```python
from build123d import *

# Parameters (mm, degrees)
PAD_DEPTH       = 28.5
SKETCH001_R     = 14.25
POCKET_DEPTH    = 18.5
SKETCH002_R     = 1.375
POCKET001_DEPTH = 12
SKETCH003_W     = 4
SKETCH003_H     = 10.5
POCKET002_DEPTH = 8
SKETCH004_R     = 1.75
POCKET003_DEPTH = 8
SKETCH005_R     = 3.25
POCKET004_DEPTH = 6
SKETCH006_R     = 1.375
POCKET005_DEPTH = 10
SKETCH007_R     = 1.375
POCKET006_DEPTH = 10


with BuildPart() as recess_pocket:
    # Sketch → Pad (new body)
    with BuildSketch(Plane.YZ):
        with BuildLine():
            ThreePointArc((2.722222, 19.699888), (-1.166667, 20.799832), (-3.5, 17.5))
            Line((-3.5, 17.5), (-3.5, -17.5))
            ThreePointArc((-3.5, -17.5), (-1.166657, -20.799835), (2.722235, -19.699872))
            Line((2.722235, -19.699872), (4.5, -17.5))
            Line((4.5, 17.5), (4.5, -17.5))
            Line((4.5, 17.5), (2.722222, 19.699888))
        make_face()
    extrude(amount=PAD_DEPTH)

    # Sketch001 → Pocket (cut)
    with BuildSketch(Plane.YZ.offset(28.5)):
        Circle(SKETCH001_R)
    extrude(amount=-POCKET_DEPTH, mode=Mode.SUBTRACT)

    # Sketch002 → Pocket001 (cut)
    with BuildSketch(Plane.YZ.offset(28.5)):
        with Locations((0, -17.5)):
            Circle(SKETCH002_R)
        with Locations((0, 17.5)):
            Circle(SKETCH002_R)
    extrude(amount=-POCKET001_DEPTH, mode=Mode.SUBTRACT)

    # Sketch003 → Pocket002 (cut)
    with BuildSketch(Plane(origin=(0, -3.5, 0), x_dir=(0, 0, -1), z_dir=(0, -1, 0))):
        with Locations((-20, 5.25)):
            Rectangle(SKETCH003_W, SKETCH003_H)
        with Locations((20, 5.25)):
            Rectangle(SKETCH003_W, SKETCH003_H)
    extrude(amount=-POCKET002_DEPTH, mode=Mode.SUBTRACT)


with BuildPart() as bottom_screw_hole_pocket:
    # Part__Mirroring: instance of recess-pocket
    add(recess_pocket.part.mirror(Plane(origin=(0, 0, 0), x_dir=(0, -1, 0), z_dir=(1, 0, 0))))

    # Fusion: union recess-pocket
    add(recess_pocket.part)

    # Sketch004 → Pocket003 (cut)
    with BuildSketch(Plane.XZ.offset(3.5)):
        Circle(SKETCH004_R)
    extrude(amount=-POCKET003_DEPTH, mode=Mode.SUBTRACT)

    # Sketch005 → Pocket004 (cut)
    with BuildSketch(Plane.XZ.offset(3.5)):
        Circle(SKETCH005_R)
    extrude(amount=-POCKET004_DEPTH, mode=Mode.SUBTRACT)

    # Sketch006 → Pocket005 (cut)
    with BuildSketch(Plane.XY.offset(18)):
        with Locations((0, 0.5)):
            Circle(SKETCH006_R)
    extrude(amount=-POCKET005_DEPTH, mode=Mode.SUBTRACT)

    # Sketch007 → Pocket006 (cut)
    with BuildSketch(Plane(origin=(0, 0, -18), x_dir=(1, 0, 0), z_dir=(0, 0, -1))):
        with Locations((0, -0.5)):
            Circle(SKETCH007_R)
    extrude(amount=-POCKET006_DEPTH, mode=Mode.SUBTRACT)


solid = bottom_screw_hole_pocket.part
```
Can you work these out from the model? Positions are in its coordinate system, mm. A direction names the side the tool comes from. Give positions to 0.01 mm unless a question says otherwise; leave off trailing zeros. Order: outer loops, then holes, each group sorted by start corner. A loop starts at its lowest first (then second) coordinate and runs counter-clockwise, first axis right, second up. Notation, with made-up numbers: M 54.5,46 L 102.5,46 A6 cw 102.5,50 Z; hole C 37.5,-20 d1. An arc over 180 degrees is marked long. One line per item, written item: value.
1) Please list where these lines run through material, in increasing order: line 1 along X through (y, z) = (1.25, -18.5); line 2 along Z through (x, y) = (19, 0.5); line 3 along Y through (x, z) = (0, -13.5) (3 decimals).
Answer sheet:
line 1: x = -28.5 to -10.5, 10.5 to 28.5
line 2: z = -20.96 to -18.78, -16.22 to -14.24, 14.24 to 16.22, 18.78 to 20.96
line 3: y = -3.5 to -0.875, 1.875 to 4.5
2) I want a section at D-D, the plane x = 13. List the corners of the cut face in (y, z) for me, plus the area to 3 significant figures.
Answer sheet:
outline: M -3.5,-17.5 A3.5 ccw 2.72,-19.7 L 4.5,-17.5 L 4.5,-13.52 A14.25 cw -3.5,-13.81 Z; M -3.5,13.81 A14.25 cw 4.5,13.52 L 4.5,17.5 L 2.72,19.7 A3.5 ccw -3.5,17.5 Z
area: 95.2 mm^2
3) I want a section at B-B, the plane z = -9. List the corners of the cut face in (x, y) for me (3 decimals).
Answer sheet:
outline: M -10,-3.5 L 10,-3.5 L 10,4.5 L -10,4.5 Z; hole C 0,0.5 d2.75
4) We'd pull the mould along X, two halves only. Please class faces 6 (the face through (28.5, 1, -16)), 7 (the face through (1.4, 2.5, -1.4)), 8 (the face through (19.38, 0.464, -14.242)): released by +X, released by -X, zero draft, split by the parting line, or undercut.
Answer sheet:
face 6: released by +X
face 7: undercut
face 8: zero draft
5) I want a section at A-A, the plane x = 0. List the corners of the cut face in (y, z) for me (3 decimals), plus the area to 3 significant figures.
Answer sheet:
outline: M -3.5,-17.5 A3.5 ccw -3.464,-18 L -0.875,-18 L -0.875,-8 L 1.875,-8 L 1.875,-18 L 4.096,-18 L 4.5,-17.5 L 4.5,-1.75 L 2.5,-1.75 L 2.5,-3.25 L -3.5,-3.25 Z; M -3.5,3.25 L 2.5,3.25 L 2.5,1.75 L 4.5,1.75 L 4.5,17.5 L 4.096,18 L 1.875,18 L 1.875,8 L -0.875,8 L -0.875,18 L -3.464,18 A3.5 ccw -3.5,17.5 Z
area: 187 mm^2
6) On a 3-axis mill with a long thin cutter (end or side, diameter ignored), from which of +Z, -Z, +X, -X, +Y, -Y can I reach the whole of each face in a straight line? I mean faces 1 (the face through (22.584, -0.179, 18.863)), 2 (the face through (-22.584, -0.179, -16.137)), 3 (the face through (-0.1, -1.4, -18)), 4 (the face through (0, 0, -8)), 5 (the face through (-0.1, -1.4, 18)). Say none if no direction works.
Answer sheet:
face 1: +X
face 2: -X
face 3: -Z, +Y, -Y
face 4: -Z
face 5: +Z, +Y, -Y
7) For P1, Ø2.5, axis at x = 0, y = 0.5, coming from the -Z side; P2, Ø2.5, axis at x = 2, y = 0.5, coming from the +Z side; P3, Ø2.5, axis at y = -1, z = 7, coming from the +X side; P4, Ø3, axis at x = 0, z = 0, coming from the -Y side, each with a flat end and sliding along its axis, tell me the tip position at first contact or that it passes through.
Answer sheet:
P1: stops at z = -8
P2: stops at z = 18
P3: stops at x = 10
P4: passes through
8) I want a section at C-C, the plane y = -2.5. List the corners of the cut face in (x, z) for me.
Answer sheet:
outline: M -28.5,-19.95 L -10.5,-19.95 L -10.5,-18 L 10.5,-18 L 10.5,-19.95 L 28.5,-19.95 L 28.5,-14.03 L 10,-14.03 L 10,14.03 L 28.5,14.03 L 28.5,19.95 L 10.5,19.95 L 10.5,18 L -10.5,18 L -10.5,19.95 L -28.5,19.95 L -28.5,14.03 L -10,14.03 L -10,-14.03 L -28.5,-14.03 Z; hole C 0,0 d6.5
